Design review of the part built by this model. Coordinates are the model's own, in mm. A direction names the side the tool comes from. Coordinates: 2 decimals unless noted, no trailing zeros. Loops run counter-clockwise (first coordinate to the right, second up) from the corner with the lowest first, then second, coordinate; pieces in that order, holes last. Notation, with made-up numbers: (36, 10) - (45, 10) arc R16 ccw to (45, 15) - close; hole circle Ø9 at (-12, -35). An arc over 180 degrees is marked (long way). Use one line per item in the form item = value. Start each with the question number.
(1) Add section A-A (x = 3.25). State the section outline as (y, z) points, plus the area to 3 significant figures.
(2) For L1, parallel to X at y = 4.95, z = 2; L2, parallel to X at y = 5.85, z = 3.25; L3, parallel to Z at x = 0.5, y = 6.35, list the stretches that pass through material, from the lowest coordinate up.
(3) The part is to be moulded in two halves that separate along Z. For faces 1 (the face through (-5.3, 7.98, -0.1)), 2 (the face through (6.639, 5.251, -0.408)), 3 (the face through (0.42, 5.97, -8.24)), say which applies: pulls with the +Z half, pulls with the -Z half, needs draft (parallel to the pull), parting line crosses it, or undercut.
(4) Tool access review of faces 4 (the face through (-5.3, 4.02, -0.1)), 5 (the face through (-6.48, 6.82, -0.5)): name each direction out of +Z, -Z, +X, -X, +Y, -Y from which nothing blocks a thin tool from reaching the whole face with its end or side.
(5) Add section C-C (y = 7.2). State the section outline as (x, z) points.
(6) Add section D-D (z = -0.25). Count the separate pieces of the cut face and the enclosed holes in it, plus the area to 3 significant figures.
(7) Clearance check with flat-ended pins moving along their axes: pin 1 Ø1 at (x, y) = (-5.5, 5) entering from -Z; pin 2 Ø9 at (x, z) = (0.05, 0) entering from -Y; pin 3 Ø1 at (y, z) = (5.5, -1.5) entering from +X. State where each tip first meets the part, or that it passes through.
(8) Add section B-B (z = -3.75). State the section outline as (x, y) points, plus the area to 3 significant figures.
```python
from build123d import *

# Parameters (mm, degrees)
SKETCH1_R           = 25
SKETCH1_R_2         = 15
BOSS_EXTRUDE1_DEPTH = 12
SCALE1_SCALE        = 0.33


with BuildPart() as part:
    # Sketch1 → Boss-Extrude1 (new body)
    with BuildSketch(Plane(origin=(0, 0, 0), x_dir=(1, 0, 0), z_dir=(0, 1, 0))):
        with Locations(Location((0, 0, 0), (0, 0, 270))):
            Circle(SKETCH1_R)
        with Locations(Location((0, 0, 0), (0, 0, 270))):
            Circle(SKETCH1_R_2, mode=Mode.SUBTRACT)
    extrude(amount=BOSS_EXTRUDE1_DEPTH)

    # Sketch2 → Cut-Revolve1 (revolve, cut)
    with BuildSketch(Plane.XY, mode=Mode.PRIVATE) as cut_revolve1_sk:
        Polygon((30, 8.5), (30, 6), (-30, 6), (-30, 9), align=None)
    revolve(cut_revolve1_sk.sketch.rotate(Axis((30, 6, 0), (-1, 0, 0)), 133.934111216), axis=Axis((30, 6, 0), (-1, 0, 0)), mode=Mode.SUBTRACT)


with BuildPart() as part_1:
    # Scale1: scaled about (0.080152948, 5.999999597, -1.2051e-05)
    add(part.part.scale(SCALE1_SCALE).moved(Location((0.053702475, 4.01999973, -8.074e-06))))


solid = part_1.part
```
Computed values:
q1.outline = (4.02, -7.61) - (7.98, -7.61) - (7.98, -3.78) - (4.02, -3.78) - close; (4.02, 3.78) - (7.98, 3.78) - (7.98, 7.61) - (4.02, 7.61) - close
q1.area = 30.3 mm^2
q2.L1 = -7.95 to -4.47, 4.58 to 8.06
q2.L2 = -7.53 to -3.68, 3.79 to 7.64
q2.L3 = -8.24 to -4.93, 4.93 to 8.24
q3.face_1 = needs draft
q3.face_2 = undercut
q3.face_3 = parting line crosses it
q4.face_4 = +Z, -Z, +X, -X, -Y
q4.face_5 = -X
q5.outline = circle Ø16.5 at (0.05, 0); hole circle Ø9.9 at (0.05, 0)
q6.separate_pieces = 4
q6.enclosed_holes = 0
q6.area = 14.6 mm^2
q7.pin_1 = -6.52
q7.pin_2 = through
q7.pin_3 = 8.24
q8.outline = (-7.29, 4.02) - (-3.18, 4.02) - (-3.18, 7.98) - (-7.29, 7.98) - close; (3.28, 4.02) - (7.4, 4.02) - (7.4, 7.98) - (3.28, 7.98) - close
q8.area = 32.6 mm^2
